Part model, mm, in its own coordinate system. Face numbers are marked on the shaded views. Coordinates: 2 decimals unless noted, no trailing zeros. Order: outer loops, then holes, each group sorted by start corner. A loop starts at its lowest first (then second) coordinate and runs counter-clockwise, first axis right, second up. Notation, with made-up numbers: (-13, 87.25) - (39, 87.25) arc R20 ccw to (39, 114.25) - close; hole circle Ø1 at (82, -11.5). An arc over 180 degrees is marked (long way). Use a Markdown table: item, result. Add a question column.
1) Saw through at C-C on z = 0. List the corners of the cut face in (x, y) (3 decimals).
2) Saw through at D-D on y = 10.5. List the corners of the cut face in (x, z) (3 decimals), then the cut area to 3 significant figures.
3) Drop flat-ended pins along their axis: P1, Ø12, axis at y = -0.5, z = 0.5, coming from the -X side; P2, Ø1, axis at x = -1, z = -8, coming from the +Y side; P3, Ø1, axis at x = 1, y = -5, coming from the +Z side. Give the stop position or say it passes through.
4) Two-plate mould, pull along Z, no slides. Class the marked faces 1, 2 and 3: +Z half, -Z half, draft (parallel to the pull), parting line (faces both ways), or undercut.
5) Wall check: L1, parallel to Z at x = -0.45, y = 2 (3 decimals); L2, parallel to Y at x = 0.35, z = 0 (3 decimals); L3, parallel to Y at x = -1.15, z = -1.25. Give the ranges that are in metal, low to high. Write a range as [from, to].
6) Saw through at B-B on y = 0. List the corners of the cut face in (x, z) (3 decimals), then the cut area to 3 significant figures.
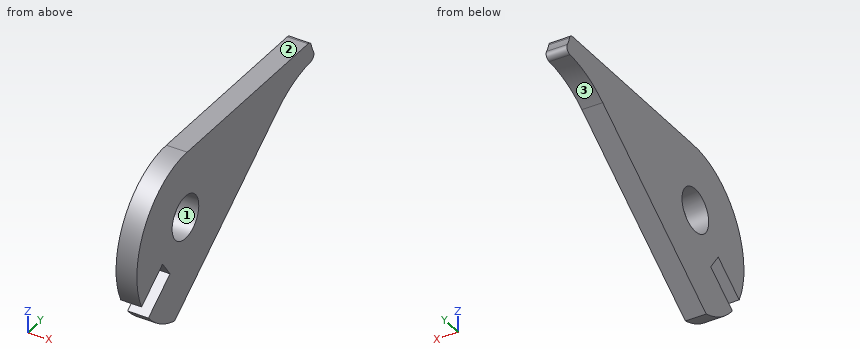
```python
from build123d import *

# Parameters (mm, degrees)
BOSS_EXTRUDE1_DEPTH = 1.524
SKETCH2_R           = 3.175
CUT_EXTRUDE1_DEPTH  = 4.048
CUT_EXTRUDE2_DEPTH  = 4.048


with BuildPart() as part:
    # Sketch1 → Boss-Extrude1 (new body, symmetric)
    with BuildSketch(Plane(origin=(0, 0, 0), x_dir=(0, 0, -1), z_dir=(1, 0, 0))):
        with BuildLine():
            Line((-9.525, 29.203153615), (-9.525, 0.413383537))
            ThreePointArc((-9.525, 0.413383537), (0.953114694, -11.479629163), (14.071488999, -2.58339995))
            Line((14.071488999, -2.58339995), (-3.690440969, 22.065775388))
            ThreePointArc((-3.690440969, 22.065775388), (-5.633424794, 25.762785311), (-6.474725684, 29.85366313))
            ThreePointArc((-6.474725684, 29.85366313), (-6.888835567, 30.502157859), (-7.658237218, 30.494842983))
            ThreePointArc((-7.658237218, 30.494842983), (-8.281558069, 30.191808808), (-8.938016281, 29.969499991))
            ThreePointArc((-8.938016281, 29.969499991), (-9.361392761, 29.685812049), (-9.525, 29.203153615))
        make_face()
    extrude(amount=BOSS_EXTRUDE1_DEPTH, both=True)

    # Sketch2 → Cut-Extrude1 (cut, through all)
    with BuildSketch(Plane(origin=(1.524, 0, 0), x_dir=(0, 0, -1), z_dir=(1, 0, 0))):
        Circle(SKETCH2_R)
    extrude(amount=-CUT_EXTRUDE1_DEPTH, mode=Mode.SUBTRACT)

    # Sketch3 → Cut-Extrude2 (cut, through all)
    with BuildSketch(Plane(origin=(1.524, 0, 0), x_dir=(0, 0, -1), z_dir=(1, 0, 0))):
        with BuildLine():
            Line((3.926398482, -5.448872099), (7.531186188, -10.451427812))
            ThreePointArc((7.531186188, -10.451427812), (8.873585882, -9.717582903), (10.111597952, -8.818755111))
            Line((10.111597952, -8.818755111), (6.399264057, -3.66695183))
            Line((6.399264057, -3.66695183), (3.926398482, -5.448872099))
        make_face()
    extrude(amount=-CUT_EXTRUDE2_DEPTH, mode=Mode.SUBTRACT)


solid = part.part
```
Results are:
| question | item | result |
|---|---|---|
| 1 | outline | (-1.524, -11.319) - (1.524, -11.319) - (1.524, -3.175) - (-1.524, -3.175) - close; (-1.524, 3.175) - (1.524, 3.175) - (1.524, 16.944) - (-1.524, 16.944) - close |
| 2 | outline | (-1.524, -4.644) - (1.524, -4.644) - (1.524, 9.525) - (-1.524, 9.525) - close |
| 2 | area | 43.2 mm2 |
| 3 | P1 | x = -1.52 |
| 3 | P2 | y = 6.54 |
| 3 | P3 | z = 8.47 |
| 4 | face 1 | undercut |
| 4 | face 2 | +Z half |
| 4 | face 3 | -Z half |
| 5 | L1 | [-10.769, -2.466], [2.466, 9.525] |
| 5 | L2 | [-11.319, -3.175], [3.175, 16.944] |
| 5 | L3 | [-11.51, -2.92], [2.92, 15.21] |
| 6 | outline | (-1.524, -12.21) - (1.524, -12.21) - (1.524, -3.175) - (-1.524, -3.175) - close; (-1.524, 3.175) - (1.524, 3.175) - (1.524, 9.518) - (-1.524, 9.518) - close |
| 6 | area | 46.9 mm2 |
